```python
from build123d import *

# Parameters (mm, degrees)
F0_W      = 101
F0_H      = 36
F0_W_2    = 95.5
F0_H_2    = 27.5
F0_W_3    = 87.5
F0_H_3    = 19.5
F1_DEPTH  = 4
F1_FACE_W = 101
F1_FACE_H = 36
F2_W      = 95.5
F2_H      = 27.5
F2_W_2    = 87.5
F2_H_2    = 19.5
F3_DEPTH  = 4
F5_D      = 5
F5_DEPTH  = 6
F5_TIP    = 1.5021515476


with BuildPart() as f1:
    # F0 (on Front) → F1 (new body)
    with BuildSketch(Plane.XZ):
        Rectangle(F0_W, F0_H)
        Rectangle(F0_W_2, F0_H_2, mode=Mode.SUBTRACT)
        Rectangle(F0_W_2, F0_H_2)
        Rectangle(F0_W_3, F0_H_3, mode=Mode.SUBTRACT)
        Rectangle(F0_W_3, F0_H_3)
    extrude(amount=F1_DEPTH)

    # F1_face (on face) + F2 (on Front) → F3 (join)
    with BuildSketch(Plane.XZ.offset(4)):
        Rectangle(F1_FACE_W, F1_FACE_H)
    with BuildSketch(Plane.XZ):
        Rectangle(F2_W, F2_H)
        Rectangle(F2_W_2, F2_H_2, mode=Mode.SUBTRACT)
    extrude(amount=-F3_DEPTH)

    # F5
    with Locations(Plane(origin=(0, 0, 0), x_dir=(1, 0, 0), z_dir=(0, 1, 0))):
        with Locations((-40.1297956705, -7.1705272421)):
            Hole(F5_D / 2, depth=F5_DEPTH)
            with Locations((0, 0, -(F5_DEPTH + F5_TIP / 2))):  # 118° drill point
                Cone(0, F5_D / 2, F5_TIP, mode=Mode.SUBTRACT)


solid = f1.part
```
Input: part model. Units: mm. Frame: model coordinates. A direction names the side the tool comes from. Give positions to 0.01 mm unless a question says otherwise; leave off trailing zeros. Loops run counter-clockwise (first coordinate to the right, second up) from the corner with the lowest first, then second, coordinate; pieces in that order, holes last.
1) Section query D-D on z = 11.5. Return the cut outline in (x, y).
A:
outline: (-50.5, -4) - (50.5, -4) - (50.5, 0) - (47.75, 0) - (47.75, 4) - (-47.75, 4) - (-47.75, 0) - (-50.5, 0) - close
2) Section query A-A on y = 1.75. Return the cut outline in (x, z), and give its area (3 significant figures).
A:
outline: (-47.75, -13.75) - (47.75, -13.75) - (47.75, 13.75) - (-47.75, 13.75) - close; hole (-43.75, -9.75) - (43.75, -9.75) - (43.75, 9.75) - (-43.75, 9.75) - close
area: 920 mm2
3) Line query: L1, parallel to X at y = 3.75, z = 3; L2, parallel to Z at x = 12, y = 0.75; L3, parallel to Y at x = 21.5, z = -14. Output: solid intervals per line, ascending.
A:
L1: x = -47.75 to -43.75, 43.75 to 47.75
L2: z = -13.75 to -9.75, 9.75 to 13.75
L3: y = -4 to 0
4) Contact query for flat-ended pins moving along their axis: pin 1 (1 mm diameter, centred on x = 35, y = 2.5, fed in from -Z); pin 2 (4.5 mm diameter, centred on y = 2.5, z = 5, fed in from -X); pin 3 (2 mm diameter, centred on y = 2.5, z = -1.5, fed in from +X). Output: stop coordinate, or through.
A:
pin 1: stops at z = -13.75
pin 2: stops at x = -47.75
pin 3: stops at x = 47.75
5) Mould query, pull axis X, two halves, no side actions, for faces 5 (the flat face through (-1, 0, 0)), 6 (the flat face through (-1, -2, -18)), 7 (the flat face through (47.75, 2, 0)). Classes: released by +X, released by -X, zero draft, split by the parting line, or undercut.
A:
face 5: undercut
face 6: zero draft
face 7: released by +X
6) Section query C-C on x = -31.5. Return the cut outline in (y, z).
A:
outline: (-4, -18) - (0, -18) - (0, -13.75) - (4, -13.75) - (4, -9.75) - (0, -9.75) - (0, 9.75) - (4, 9.75) - (4, 13.75) - (0, 13.75) - (0, 18) - (-4, 18) - close
7) Section query B-B on z = 6. Return the cut outline in (x, y).
A:
outline: (-50.5, -4) - (-42.34, -4) - (-42.34, 0) - (-43.75, 0) - (-43.75, 4) - (-47.75, 4) - (-47.75, 0) - (-50.5, 0) - close; (-37.92, -4) - (50.5, -4) - (50.5, 0) - (47.75, 0) - (47.75, 4) - (43.75, 4) - (43.75, 0) - (-37.92, 0) - close
8) Reachability of faces 1 (the flat face through (-1, 2, 13.75)), 2 (the flat face through (-43.75, 2, 0)), 3 (the flat face through (-47.75, 2, 0)), 4 (the flat face through (-1, 2, -13.75)) from +Z, -Z, +X, -X, +Y, -Y: full face, straight path, thin tool, end or side. Return the list, or none.
A:
face 1: +Z, +X, -X, +Y
face 2: +Y
face 3: +Z, -Z, -X, +Y
face 4: -Z, +X, -X, +Y
